Study the drawing (mm; zero at the part's minimum x, y, z) and answer. A direction names the side the tool comes from. Round coordinates to 2 decimals unless told otherwise and drop trailing zeros. Order: outer loops, then holes, each group sorted by start corner. A loop starts at its lowest first (then second) coordinate and runs counter-clockwise, first axis right, second up. Notation, with made-up numbers: (24, 12) - (64, 12) arc R10 cw to (64, 30) - close; hole circle Ø10 at (39, 73.25). An arc over 180 degrees is marked (long way). Use one line per item in the form item = value. Start each with the question number.
Q1. The part is cut by section D-D on x = 26.7. Determine the outline of the cut face in (y, z), plus the area to 3 significant figures.
Q2. The part is cut by section B-B on y = 12. Determine the outline of the cut face in (x, z), plus the area to 3 significant figures.
Q3. Given P1, Ø2, axis at x = 12.5, z = 26, coming from the +Y side; P2, Ø12, axis at x = 15.5, y = 19, coming from the +Z side; P3, Ø8, axis at x = 4.5, y = 15, coming from the +Z side, each flat-ended and moving along its own axis, determine where each tip first touches the part or whether it passes through.
Q4. Find the intervals of material crossed by line 1 (Z direction, x = 17.85, y = 3.15); line 2 (Y direction, x = 26.7, z = 1.8); line 3 (X direction, y = 6, z = 14), in increasing order. Write a range as [from, to].
Q5. The part is cut by section C-C on z = 23. Determine the outline of the cut face in (x, y), plus the area to 3 significant figures.
Q6. For a pull along Y with two mould halves and no side action, classify the marked faces 3, 4, 5 and 6 as +Y half, -Y half, draft (parallel to the pull), parting line (faces both ways), or undercut.
Q7. The part is cut by section A-A on x = 17.85. Determine the outline of the cut face in (y, z), plus the area to 3 significant figures.
Q8. Which of the six approach directions +Z, -Z, +X, -X, +Y, -Y give full straight-line access (tool end or side, diameter ignored) to the marked faces 1 and 2?
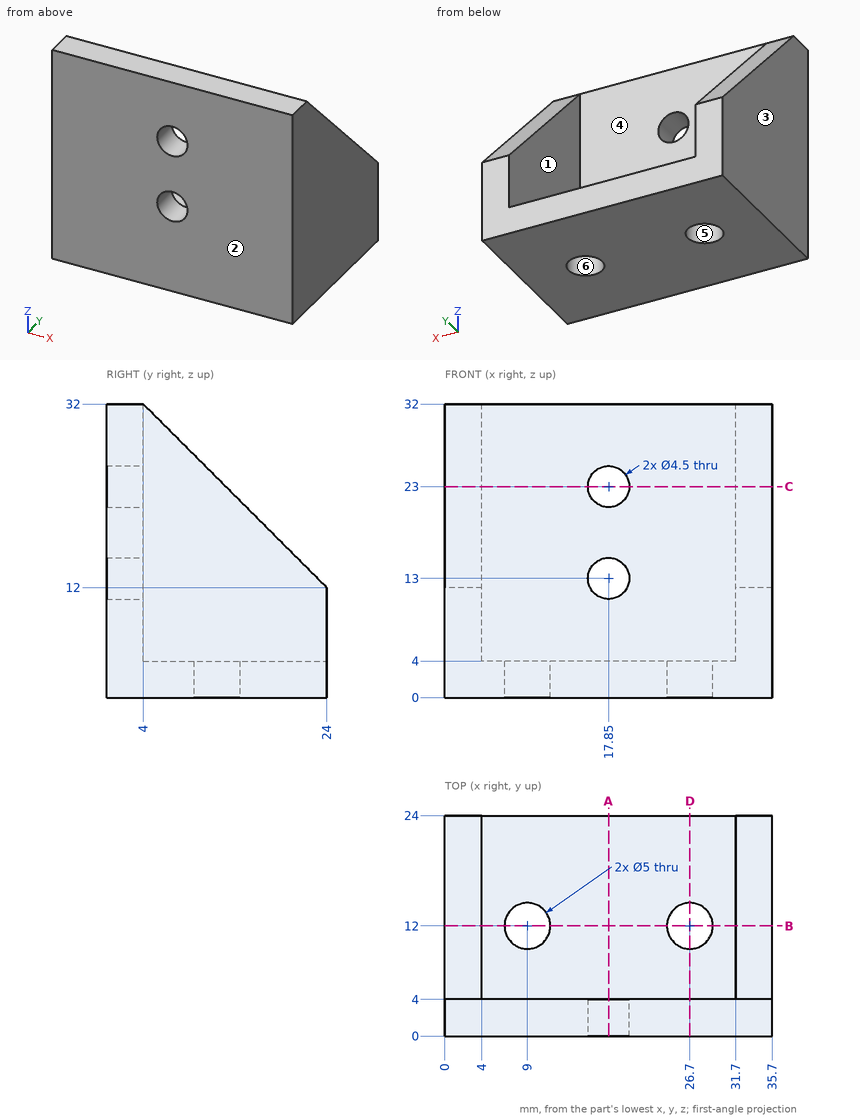
Found:
q1.outline = (0, 0) - (9.5, 0) - (9.5, 4) - (4, 4) - (4, 32) - (0, 32) - close; (14.5, 0) - (24, 0) - (24, 4) - (14.5, 4) - close
q1.area = 188 mm²
q2.outline = (0, 0) - (6.5, 0) - (6.5, 4) - (4, 4) - (4, 24) - (0, 24) - close; (11.5, 0) - (24.2, 0) - (24.2, 4) - (11.5, 4) - close; (29.2, 0) - (35.7, 0) - (35.7, 24) - (31.7, 24) - (31.7, 4) - (29.2, 4) - close
q2.area = 263 mm²
q3.P1 = 4
q3.P2 = 4
q3.P3 = 24.97
q4.line_1 = [0, 10.75], [15.25, 20.75], [25.25, 32]
q4.line_2 = [0, 9.5], [14.5, 24]
q4.line_3 = [0, 4], [31.7, 35.7]
q5.outline = (0, 0) - (15.6, 0) - (15.6, 4) - (4, 4) - (4, 13) - (0, 13) - close; (20.1, 0) - (35.7, 0) - (35.7, 13) - (31.7, 13) - (31.7, 4) - (20.1, 4) - close
q5.area = 197 mm²
q6.face_3 = draft
q6.face_4 = +Y half
q6.face_5 = undercut
q6.face_6 = undercut
q7.outline = (0, 0) - (24, 0) - (24, 4) - (4, 4) - (4, 10.75) - (0, 10.75) - close; (0, 15.25) - (4, 15.25) - (4, 20.75) - (0, 20.75) - close; (0, 25.25) - (4, 25.25) - (4, 32) - (0, 32) - close
q7.area = 172 mm²
q8.face_1 = +Z, +Y
q8.face_2 = +Z, -Z, +X, -X, -Y
